Can you work these out from the drawing? Everything is in mm from the part's minimum corner. Give positions to 0.01 mm unless a question says otherwise; leave off trailing zeros. Write each loop counter-clockwise with the first axis right and the second up, starting at its lowest first coordinate (ties: lowest second). Pieces come first, ordered by that corner, then holes. Notation, with made-up numbers: (8, -15.75) - (22, -15.75) arc R19 ccw to (22, 3.25) - close; hole circle Ø8 at (-2, 19). An arc over 180 degrees is marked (long way). Use a Markdown table: item, result.
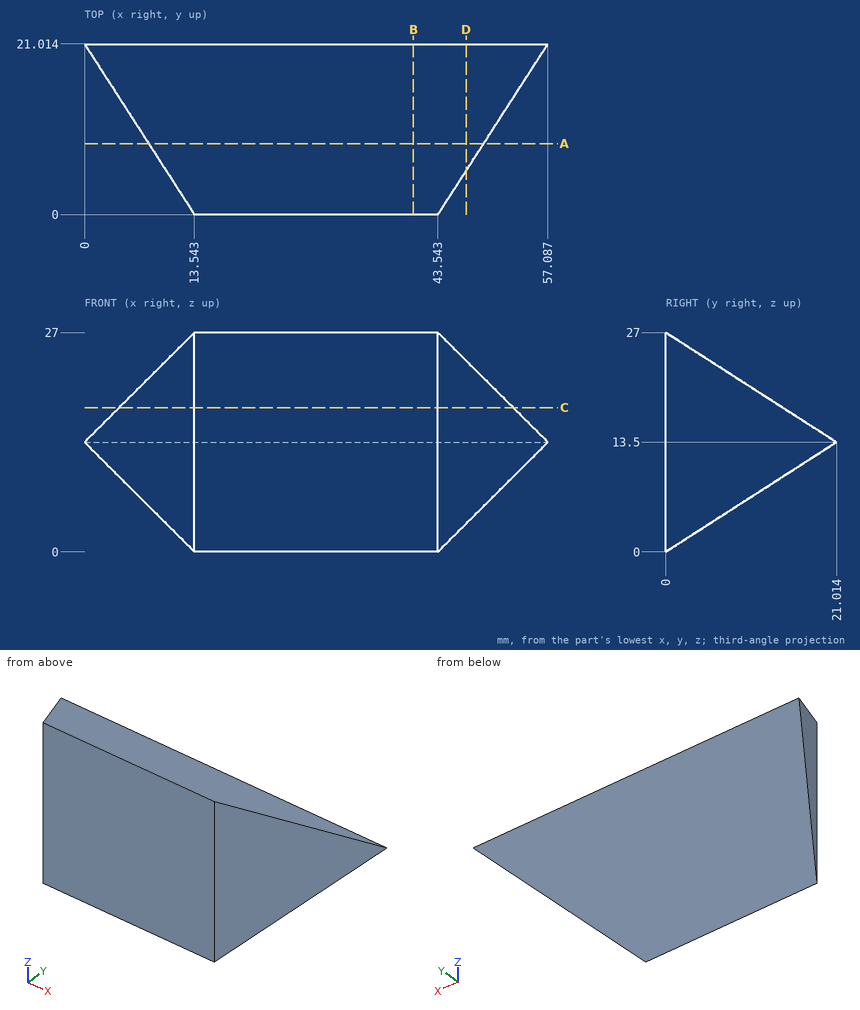
Item 1: If we section it at B-B, the plane x = 40.5: Write out the boundary of the cut face in (y, z).
Values:
| item | result |
|---|---|
| outline | (0, 0) - (21.01, 13.5) - (0, 27) - close |
Item 2: If we section it at A-A, the plane y = 8.75: Write out the boundary of the cut face in (x, z).
Values:
| item | result |
|---|---|
| outline | (7.9, 5.62) - (49.18, 5.62) - (49.18, 21.38) - (7.9, 21.38) - close |
Item 3: Will these pins go through, and if not, where does the flat tip stop? pin 1 Ø2 at (x, z) = (14, 10) entering from +Y; pin 2 Ø10 at (y, z) = (3.5, 7.5) entering from +X; pin 3 Ø3 at (x, y) = (14.5, 11) entering from +Z; pin 4 Ø1.5 at (x, z) = (16, 7) entering from -Y.
Values:
| item | result |
|---|---|
| pin 1 | stops at y = 17.12 |
| pin 2 | stops at x = 49.02 |
| pin 3 | stops at z = 20.9 |
| pin 4 | stops at y = 0 |
Item 4: I need wall thicknesses on line 1 along Z through (x, y) = (3, 17); line 2 along Z through (x, y) = (17, 2.75) (1 decimal); line 3 along Y through (x, z) = (26.5, 25.5) (1 decimal). Which ranges of each line are inside material? Lowest first, please. Write a range as [from, to].
Values:
| item | result |
|---|---|
| line 1 | z = [10.92, 16.08] |
| line 2 | z = [1.8, 25.2] |
| line 3 | y = [0, 2.3] |
Item 5: If we section it at C-C, the plane z = 17.75: Write out the boundary of the cut face in (x, y).
Values:
| item | result |
|---|---|
| outline | (4.26, 14.4) - (13.54, 0) - (43.54, 0) - (52.82, 14.4) - close |
Item 6: If we section it at D-D, the plane x = 47: Write out the boundary of the cut face in (y, z) (1 decimal).
Values:
| item | result |
|---|---|
| outline | (5.4, 3.4) - (21, 13.5) - (5.4, 23.6) - close |
